from build123d import *

# Parameters (mm, degrees)
SALIENTE_EXTRUIR1_DEPTH      = 220
SALIENTE_EXTRUIR1_DEPTH_BACK = 220
CROQUIS1_R                   = 5
CORTAR_EXTRUIR1_DEPTH        = 221.113607031
CORTAR_EXTRUIR1_DEPTH_BACK   = 221.113607031
CROQUIS6_R                   = 58.510219283


with BuildPart() as part:
    # Croquis1 → Saliente-Extruir1 (new, two sides: drawn at the far end of the back side and taken through both)
    with BuildSketch(Plane.XY.offset(-SALIENTE_EXTRUIR1_DEPTH_BACK)):
        Circle(CROQUIS1_R)
    extrude(amount=SALIENTE_EXTRUIR1_DEPTH + SALIENTE_EXTRUIR1_DEPTH_BACK)

    # Croquis5 → Perforador para roscar para macho de roscar para M5x0.81 (revolve, cut)
    with BuildSketch(Plane(origin=(0, 0, 220), x_dir=(0, -1, 0), z_dir=(1, 0, 0))):
        Polygon((0, 0), (0, 41.2618073), (2.1, 40), (2.1, 0), align=None)
    perforador_para_roscar_para_macho_de_ros = revolve(axis=Axis((0, 0, 226.35), (0, 0, -1)), mode=Mode.SUBTRACT)

    # Simetría2: Perforador para roscar para macho de roscar para M5x0.81 across plane
    add(perforador_para_roscar_para_macho_de_ros.mirror(Plane.XY), mode=Mode.SUBTRACT)

    # Croquis6 → Cortar-Extruir1 (cut, two sides: drawn at the far end of the back side and taken through both)
    with BuildSketch(Plane(origin=(0, 0, 0), x_dir=(1, 0, 0), z_dir=(0, 1, 0)).offset(-CORTAR_EXTRUIR1_DEPTH_BACK)):
        with Locations((-58.510219283, 0)):
            Circle(CROQUIS6_R)
    extrude(amount=CORTAR_EXTRUIR1_DEPTH + CORTAR_EXTRUIR1_DEPTH_BACK, mode=Mode.SUBTRACT)


solid = part.part
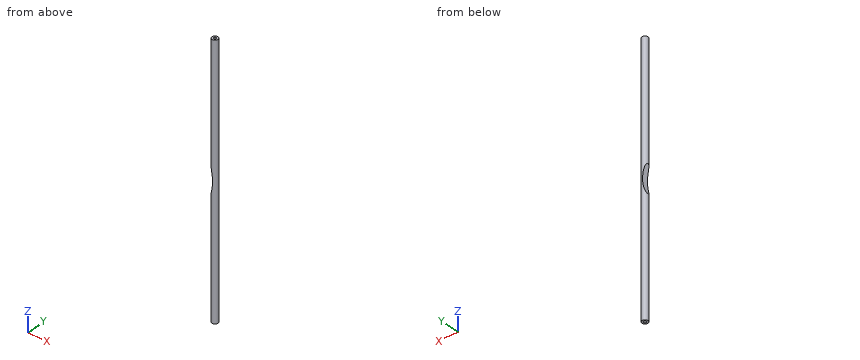
The listing builds one solid part. Answer for the finished solid, in the listing's coordinates (mm). Round coordinates to 2 decimals unless told otherwise and drop trailing zeros. Write each loop counter-clockwise with the first axis right and the second up, starting at its lowest first coordinate (ties: lowest second). Pieces come first, ordered by that corner, then holes. Notation, with made-up numbers: M 73.5,61 L 113.5,61 A15 cw 113.5,65 Z; hole C 75.5,51 d8. An arc over 180 degrees is marked long. Write each question's results on one line, items separated by ' | '. Start each with the question number.
Item 1: A cutting plane is placed at A-A on z = -64. Write down the section's boundary in (x, y), and give its area (3 significant figures).
Item 2: A cutting plane is placed at B-B on z = 10. Write down the section's boundary in (x, y), and give its area (3 significant figures).
Item 3: Straight lines are drawn through the part: L1, parallel to Y at x = 0, z = -205; L2, parallel to X at y = -0.75, z = -58. For each, find the intervals that lie inside material, in ascending order. Write a range as [from, to].
Item 4: Flat-ended cylindrical pins translate along their axes: pin 1 Ø4 at (x, y) = (0, 0) entering from -Z; pin 2 Ø5 at (y, z) = (-1.5, -113) entering from +X; pin 3 Ø1.5 at (x, z) = (-1.5, -120) entering from +Y; pin 4 Ø4 at (x, y) = (0, 0) entering from +Z. Find the tip coordinate at first contact, or state that the pin passes through.
Check sheet entries:
1) outline: C 0,0 d10 | area: 78.5 mm²
2) outline: M -0.86,-4.93 A5 ccw long -0.86,4.93 Z | area: 47.8 mm²
3) L1: [-5, -2.1], [2.1, 5] | L2: [-4.94, 4.94]
4) pin 1: z = -179.94 | pin 2: x = 5 | pin 3: y = 4.94 | pin 4: z = 179.94
